```python
from build123d import *

# Parameters (mm, degrees)
SKETCH1_R           = 7
BOSS_EXTRUDE1_DEPTH = 4
SKETCH2_W           = 4.5
SKETCH2_H           = 8
BOSS_EXTRUDE2_DEPTH = 10
FILLET2_R           = 0.5


with BuildPart() as part:
    # Sketch1 → Boss-Extrude1 (new body)
    with BuildSketch(Plane(origin=(0, 0, 0), x_dir=(1, 0, 0), z_dir=(0, 1, 0))):
        with Locations(Location((0, 0, 0), (0, 0, 270))):
            Circle(SKETCH1_R)
    extrude(amount=BOSS_EXTRUDE1_DEPTH)

    # Sketch2 → Boss-Extrude2 (add)
    with BuildSketch(Plane(origin=(0, 4, 0), x_dir=(1, 0, 0), z_dir=(0, 1, 0))):
        Rectangle(SKETCH2_W, SKETCH2_H)
    extrude(amount=BOSS_EXTRUDE2_DEPTH)

    # Fillet2
    fillet2_edges = [part.edges().sort_by_distance(p)[0] for p in [
        (-2.25, 4, 0),
        (0, 4, 4),
        (2.25, 4, 0),
        (0, 4, -4),
    ]]
    fillet(fillet2_edges, radius=FILLET2_R)


solid = part.part
```
Verification items for the finished model (mm, model axes). A direction names the side the tool comes from. Give positions to 0.01 mm unless a question says otherwise; leave off trailing zeros. Loops run counter-clockwise (first coordinate to the right, second up) from the corner with the lowest first, then second, coordinate; pieces in that order, holes last.
1. Set-up check for faces 1 (the flat face through (0, 9, -4)), 2 (the flat face through (2.25, 9, 0)), 3 (the flat face through (-3, 4, 0)), 4 (the flat face through (0, 9, 4)): record each of +Z, -Z, +X, -X, +Y, -Y from which the full face is reachable in a straight line by a thin tool's end or side.
2. Section check C-C, the plane y = 8.5. Enter the section's corners in (x, z), then the cut area to 3 significant figures.
3. Section check A-A, the plane z = 0. Enter the section's corners in (x, y), then the cut area to 3 significant figures.
4. Go/stop test with flat-tipped pins: pin 1 Ø1.3 at (x, y) = (-0.5, 11) entering from +Z; pin 2 Ø4 at (y, z) = (7.5, -1.5) entering from -X; pin 3 Ø8 at (y, z) = (6, -5) entering from -X. Record where each tip stops, or that it passes through.
5. Section check D-D, the plane y = 4.25. Enter the section's corners in (x, z).
6. Thickness scan on line 1 (Z direction, x = 1.25, y = 7.25); line 2 (Y direction, x = -5.25, z = 2); line 3 (X direction, y = 4.75, z = 3). Record the ranges inside material, lowest first.
7. Section check B-B, the plane x = 0.5. Enter the section's corners in (y, z), then the cut area to 3 significant figures.
Geometry says:
1. face 1: -Z, +X, -X, +Y
1. face 2: +Z, -Z, +X, +Y
1. face 3: +Y
1. face 4: +Z, +X, -X, +Y
2. outline: (-2.25, -4) - (2.25, -4) - (2.25, 4) - (-2.25, 4) - close
2. area: 36.0 mm2
3. outline: (-7, 0) - (7, 0) - (7, 4) - (2.75, 4) arc R0.5 cw to (2.25, 4.5) - (2.25, 14) - (-2.25, 14) - (-2.25, 4.5) arc R0.5 cw to (-2.75, 4) - (-7, 4) - close
3. area: 101 mm2
4. pin 1: stops at z = 4
4. pin 2: stops at x = -2.25
4. pin 3: stops at x = -6.83
5. outline: (-2.32, -4.07) - (2.32, -4.07) - (2.32, 4.07) - (-2.32, 4.07) - close
6. line 1: z = -4 to 4
6. line 2: y = 0 to 4
6. line 3: x = -2.25 to 2.25
7. outline: (0, -6.98) - (4, -6.98) - (4, -4.5) arc R0.5 cw to (4.5, -4) - (14, -4) - (14, 4) - (4.5, 4) arc R0.5 cw to (4, 4.5) - (4, 6.98) - (0, 6.98) - close
7. area: 136 mm2
